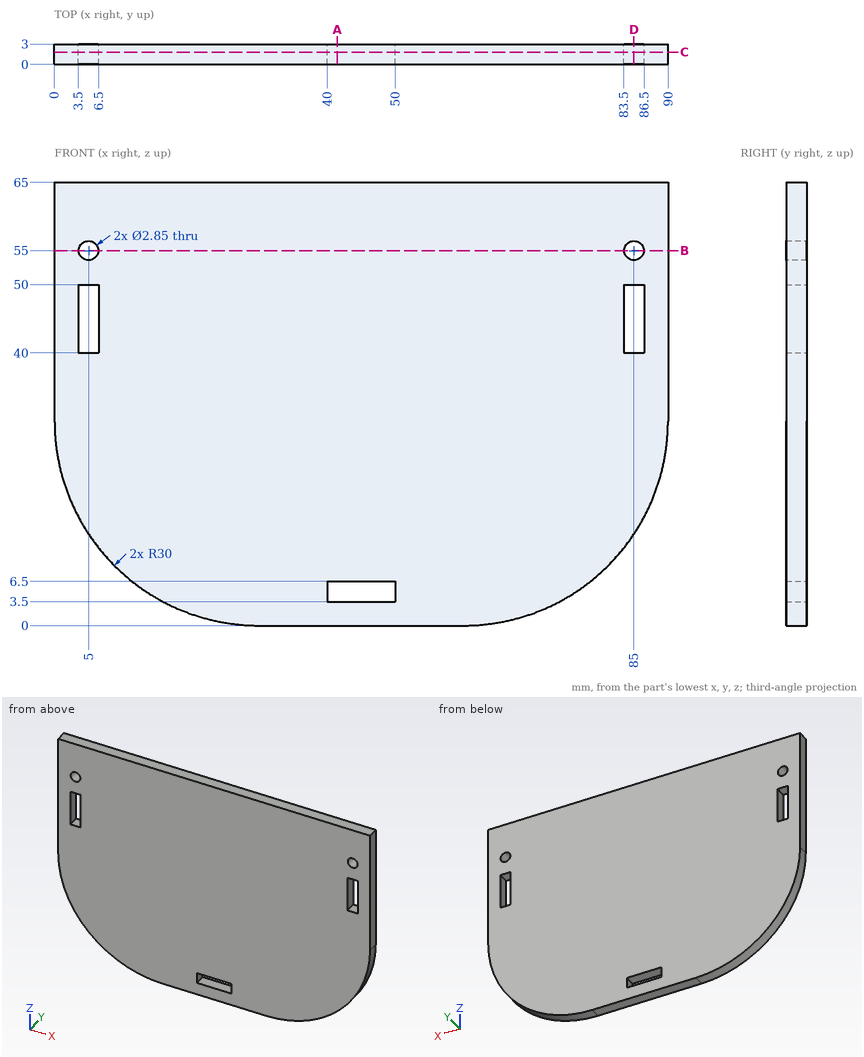
Design review of the part shown in the three views and the two pictorial views. Dimensions are in mm from the part's minimum x, y and z. Give positions to 0.01 mm unless a question says otherwise; leave off trailing zeros. Loops run counter-clockwise (first coordinate to the right, second up) from the corner with the lowest first, then second, coordinate; pieces in that order, holes last. Notation, with made-up numbers: (62.25, 42.5) - (88.25, 42.5) arc R18 ccw to (88.25, 76.5) - close; hole circle Ø10 at (-20, 31.5). An arc over 180 degrees is marked (long way). Write item = value, one per line.
1) Take a section at D-D on x = 85. State the section outline as (y, z) points (3 decimals), and give its area (3 significant figures).
Result sheet:
outline = (0, 13.417) - (3, 13.417) - (3, 40) - (0, 40) - close; (0, 50) - (3, 50) - (3, 53.575) - (0, 53.575) - close; (0, 56.425) - (3, 56.425) - (3, 65) - (0, 65) - close
area = 116 mm2
2) Take a section at B-B on z = 55. State the section outline as (x, y) points (3 decimals), and give its area (3 significant figures).
Result sheet:
outline = (0, 0) - (3.575, 0) - (3.575, 3) - (0, 3) - close; (6.425, 0) - (83.575, 0) - (83.575, 3) - (6.425, 3) - close; (86.425, 0) - (90, 0) - (90, 3) - (86.425, 3) - close
area = 253 mm2
3) Take a section at C-C on y = 1.8. State the section outline as (x, z) points (3 decimals), and give its area (3 significant figures).
Result sheet:
outline = (0, 30) arc R30 ccw to (30, 0) - (60, 0) arc R30 ccw to (90, 30) - (90, 65) - (0, 65) - close; hole (3.5, 40) - (6.5, 40) - (6.5, 50) - (3.5, 50) - close; hole circle Ø2.85 at (5, 55); hole (40, 3.5) - (50, 3.5) - (50, 6.5) - (40, 6.5) - close; hole (83.5, 40) - (86.5, 40) - (86.5, 50) - (83.5, 50) - close; hole circle Ø2.85 at (85, 55)
area = 5,360 mm2
4) To check wall thickness, follow line 1 (X direction, y = 2.2, z = 55) (3 decimals); line 2 (X direction, y = 2.3, z = 6); line 3 (Z direction, x = 81, y = 1.65). State the ranges of each line that lie inside material, in increasing order.
Result sheet:
line_1 = 0 to 3.575, 6.425 to 83.575, 86.425 to 90
line_2 = 12 to 40, 50 to 78
line_3 = 8.58 to 65
5) Take a section at A-A on x = 41.5. State the section outline as (y, z) points, and give its area (3 significant figures).
Result sheet:
outline = (0, 0) - (3, 0) - (3, 3.5) - (0, 3.5) - close; (0, 6.5) - (3, 6.5) - (3, 65) - (0, 65) - close
area = 186 mm2
6) Clearance check with flat-ended pins moving along their axes: pin 1 Ø4.5 at (x, z) = (5, 55) entering from -Y; pin 2 Ø1.5 at (y, z) = (2, 5) entering from +X; pin 3 Ø2.5 at (x, z) = (85, 55) entering from +Y; pin 4 Ø0.9 at (x, y) = (85, 1.5) entering from -Z. State where each tip first meets the part, or that it passes through.
Result sheet:
pin_1 = 0
pin_2 = 77.66
pin_3 = through
pin_4 = 12.76
